```python
from build123d import *

# Parameters (mm, degrees)
F0_W      = 17.8937
F0_H      = 17.4498
F0_R      = 4.953
F1_DEPTH  = 7.8994
F2_R      = 12.4968
F3_DEPTH  = 50.8
F3_FACE_R = 4.953
F4_DEPTH  = 50.8


with BuildPart() as f1:
    # F0 (on Front) → F1 (new body)
    with BuildSketch(Plane.XZ):
        Rectangle(F0_W, F0_H)
        Circle(F0_R, mode=Mode.SUBTRACT)
    extrude(amount=F1_DEPTH)

    # F2 (on Front) → F3 (join)
    with BuildSketch(Plane.XZ):
        Circle(F2_R)
    extrude(amount=-F3_DEPTH)

    # F3_face (on face) → F4 (cut)
    with BuildSketch(Plane.XZ):
        Circle(F3_FACE_R)
    extrude(amount=-F4_DEPTH, mode=Mode.SUBTRACT)


solid = f1.part
```
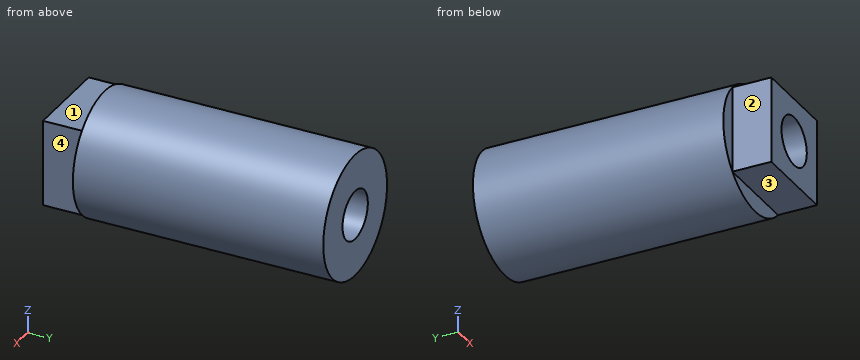
CAD build for the part. Positions are in the model's coordinates, mm. Face numbers are marked on the shaded views. A direction names the side the tool comes from. Round coordinates to 2 decimals unless told otherwise and drop trailing zeros. Order: outer loops, then holes, each group sorted by start corner. A loop starts at its lowest first (then second) coordinate and runs counter-clockwise, first axis right, second up. Notation, with made-up numbers: (47, 48.25) - (85, 48.25) arc R32 ccw to (85, 81.25) - close; hole circle Ø6 at (48, 74.5). An arc over 180 degrees is marked (long way). Use CSV: the item, a comma, the result in double quotes. Start each with the question number.
1) Tool access for the marked faces 1, 2, 3 and 4: list every direction of +Z, -Z, +X, -X, +Y, -Y with a clear straight run to the whole face (end or side of a thin tool).
2) Wall check: L1, parallel to Z at x = 0, y = 41.5; L2, parallel to Y at x = 10.75, z = 2.75; L3, parallel to X at y = 10, z = 1.75. Give the ranges that are in metal, low to high. Write a range as [from, to].
3) Saw through at B-B (z = 0). List the corners of the cut face in (x, y).
4) Saw through at D-D (z = -6.5). List the corners of the cut face in (x, y).
5) Saw through at C-C (y = 15). List the corners of the cut face in (x, z), and give its area (3 significant figures).
6) Saw through at A-A (x = 0). List the corners of the cut face in (y, z).
7) Pin check, flat tips, straight feed: pin 1 Ø2.5 at (x, y) = (4, -3) entering from -Z; pin 2 Ø1.5 at (x, y) = (4.5, 21.5) entering from +Z; pin 3 Ø1 at (x, y) = (5, 25) entering from +Z. Stop position of each tip, or through.
Values follow:
1,face 1,"+Z, +X, -X, -Y"
1,face 2,"+Z, -Z, -X, -Y"
1,face 3,"-Z, +X, -X, -Y"
1,face 4,"+Z, -Z, +X, -Y"
2,L1,"z = [-12.5, -4.95], [4.95, 12.5]"
2,L2,"y = [0, 50.8]"
2,L3,"x = [-12.37, -4.63], [4.63, 12.37]"
3,outline,"(-12.5, 0) - (-8.95, 0) - (-8.95, -7.9) - (-4.95, -7.9) - (-4.95, 50.8) - (-12.5, 50.8) - close; (4.95, -7.9) - (8.95, -7.9) - (8.95, 0) - (12.5, 0) - (12.5, 50.8) - (4.95, 50.8) - close"
4,outline,"(-10.67, 0) - (-8.95, 0) - (-8.95, -7.9) - (8.95, -7.9) - (8.95, 0) - (10.67, 0) - (10.67, 50.8) - (-10.67, 50.8) - close"
5,outline,"circle Ø24.99 at (0, 0); hole circle Ø9.91 at (0, 0)"
5,area,"414 mm2"
6,outline,"(-7.9, -8.72) - (0, -8.72) - (0, -12.5) - (50.8, -12.5) - (50.8, -4.95) - (-7.9, -4.95) - close; (-7.9, 4.95) - (50.8, 4.95) - (50.8, 12.5) - (0, 12.5) - (0, 8.72) - (-7.9, 8.72) - close"
7,pin 1,"stops at z = -8.72"
7,pin 2,"stops at z = 11.92"
7,pin 3,"stops at z = 11.66"
